Design review of the part built by this model. Coordinates are the model's own, in mm. A direction names the side the tool comes from. Give positions to 0.01 mm unless a question says otherwise; leave off trailing zeros. Write each loop counter-clockwise with the first axis right and the second up, starting at its lowest first coordinate (ties: lowest second). Pieces come first, ordered by that corner, then holes. Notation, with made-up numbers: M 71.25,64 L 114.25,64 A19 ccw 114.25,96 Z; hole C 74,48 d9. An arc over 180 degrees is marked long. Answer in a Markdown table with one row per item.
```python
from build123d import *

# Parameters (mm, degrees)
SKETCH1_W                             = 57.5
SKETCH1_H                             = 35.8
BASE_EXTRUSION_DEPTH                  = 0.79375
SKETCH2_R                             = 0.25
PIR_MOUNTING_HOLES_DEPTH              = 36.158249943
SKETCH3_R                             = 0.555
CONNECTOR_MOUNTING_HOLE_DEPTH         = 36.158249943
CONNECTOR_MOUNTING_HOLE_PATTERN_COUNT = 5
CONNECTOR_MOUNTING_HOLE_PATTERN_PITCH = 2.5
SKETCH4_W                             = 25
SKETCH4_H                             = 9.9
LED_DRIVER_CLEARANCE_CUT_DEPTH        = 36.158249943
LED_DRIVER_CLEARANCE_CUT_FILLETS_R    = 3
CORNER_CUTOUT_DEPTH                   = 36.158249943
SKETCH7_R                             = 1.1
MOUNTING_SCREW_HOLES_DEPTH            = 36.158249943


with BuildPart() as part:
    # Sketch1 → Base Extrusion (new body)
    with BuildSketch(Plane(origin=(0, 0, 0), x_dir=(1, 0, 0), z_dir=(0, 1, 0))):
        with Locations((-1.5, 0)):
            Rectangle(SKETCH1_W, SKETCH1_H)
    extrude(amount=BASE_EXTRUSION_DEPTH)

    # Sketch2 → PIR Mounting Holes (cut, through all)
    with BuildSketch(Plane(origin=(0, 0.79375, 0), x_dir=(1, 0, 0), z_dir=(0, 1, 0))):
        with Locations(Location((1.796051224, -1.796051224, 0), (0, 0, 270))):
            Circle(SKETCH2_R)
        with Locations(Location((1.796051224, 1.796051224, 0), (0, 0, 270))):
            Circle(SKETCH2_R)
        with Locations(Location((-1.796051224, -1.796051224, 0), (0, 0, 270))):
            Circle(SKETCH2_R)
    extrude(amount=-PIR_MOUNTING_HOLES_DEPTH, mode=Mode.SUBTRACT)

    # Sketch3 → Connector Mounting Hole (cut, through all)
    with BuildSketch(Plane(origin=(0, 0.79375, 0), x_dir=(1, 0, 0), z_dir=(0, 1, 0))):
        with Locations(Location((-25.75, 5, 0), (0, 0, 270))):
            Circle(SKETCH3_R)
    connector_mounting_hole = extrude(amount=-CONNECTOR_MOUNTING_HOLE_DEPTH, mode=Mode.SUBTRACT)

    # Connector Mounting Hole Pattern: Connector Mounting Hole ×5
    with Locations(*[(0, 0, i * CONNECTOR_MOUNTING_HOLE_PATTERN_PITCH) for i in range(1, CONNECTOR_MOUNTING_HOLE_PATTERN_COUNT)]):
        add(connector_mounting_hole, mode=Mode.SUBTRACT)

    # Sketch4 → LED Driver Clearance Cut (cut, through all)
    with BuildSketch(Plane.XZ):
        with Locations((-1.5, -12.95)):
            Rectangle(SKETCH4_W, SKETCH4_H)
    extrude(amount=-LED_DRIVER_CLEARANCE_CUT_DEPTH, mode=Mode.SUBTRACT)

    # LED Driver Clearance Cut Fillets
    led_driver_clearance_cut_fillets_edges = [part.edges().sort_by_distance(p)[0] for p in [
        (-14, 0.396875, -8),
        (11, 0.396875, -8),
    ]]
    fillet(led_driver_clearance_cut_fillets_edges, radius=LED_DRIVER_CLEARANCE_CUT_FILLETS_R)

    # Sketch5 → Corner Cutout (cut, through all)
    with BuildSketch(Plane(origin=(0, 0.79375, 0), x_dir=(1, 0, 0), z_dir=(0, 1, 0))):
        with BuildLine():
            Line((-30.25, 11), (-27.5, 11))
            ThreePointArc((-27.5, 11), (-25.697080654, 11.602192287), (-24.617964056, 13.167012113))
            Line((-24.617964056, 13.167012113), (-23.25, 17.9))
            Line((-23.25, 17.9), (-30.25, 17.9))
            Line((-30.25, 17.9), (-30.25, 11))
        make_face()
        with BuildLine():
            Line((20.25, 17.9), (21.617964056, 13.167012113))
            ThreePointArc((21.617964056, 13.167012113), (22.697080654, 11.602192287), (24.5, 11))
            Line((24.5, 11), (27.25, 11))
            Line((27.25, 11), (27.25, 17.9))
            Line((27.25, 17.9), (20.25, 17.9))
        make_face()
    corner_cutout = extrude(amount=-CORNER_CUTOUT_DEPTH, mode=Mode.SUBTRACT)

    # Corner Cut Mirror: Corner Cutout across plane
    add(corner_cutout.mirror(Plane.XY), mode=Mode.SUBTRACT)

    # Sketch7 → Mounting Screw Holes (cut, through all)
    with BuildSketch(Plane(origin=(0, 0.79375, 0), x_dir=(1, 0, 0), z_dir=(0, 1, 0))):
        with Locations(Location((-19.5, 14, 0), (0, 0, 270))):
            Circle(SKETCH7_R)
        with Locations(Location((-19.5, -14, 0), (0, 0, 270))):
            Circle(SKETCH7_R)
        with Locations(Location((16.5, -14, 0), (0, 0, 270))):
            Circle(SKETCH7_R)
        with Locations(Location((16.5, 14, 0), (0, 0, 270))):
            Circle(SKETCH7_R)
    extrude(amount=-MOUNTING_SCREW_HOLES_DEPTH, mode=Mode.SUBTRACT)


solid = part.part
```
1) For faces 4 (the face through (15.426, 0.402, 13.762)), 5 (the face through (10.1, 0.4, -8.86)), list the 3-axis set-ups (+Z, -Z, +X, -X, +Y, -Y) from which the entire face can be reached by the end or side of a thin tool; tool diameter is ignored.
Geometry says:
| item | result |
|---|---|
| face 4 | +Y, -Y |
| face 5 | -Z, +Y, -Y |
2) To check wall thickness, follow probe 1 along Z at (x, y) = (-3, 0.3); probe 2 along Z at (x, y) = (-20, 0.4); probe 3 along X at (y, z) = (0.3, -5) (3 decimals). State the ranges of each line that lie inside material, in increasing order. Write a range as [from, to].
Geometry says:
| item | result |
|---|---|
| probe 1 | [-8, 17.9] |
| probe 2 | [-17.9, -14.98], [-13.02, 13.02], [14.98, 17.9] |
| probe 3 | [-30.25, -26.305], [-25.195, 27.25] |
3) Add section C-C (z = -14). Write out the cut boundary in (x, y).
Geometry says:
| item | result |
|---|---|
| outline | M -24.38,0 L -20.6,0 L -20.6,0.79 L -24.38,0.79 Z; M -18.4,0 L -14,0 L -14,0.79 L -18.4,0.79 Z; M 11,0 L 15.4,0 L 15.4,0.79 L 11,0.79 Z; M 17.6,0 L 21.38,0 L 21.38,0.79 L 17.6,0.79 Z |
4) Add section D-D (y = 0.55). Count the separate pieces of the cut face and the enclosed holes in it, and give its area (3 significant figures).
Geometry says:
| item | result |
|---|---|
| separate pieces | 1 |
| enclosed holes | 12 |
| area | 1,630 mm^2 |
5) Add section A-A (x = 16.5). Write out the cut boundary in (y, z).
Geometry says:
| item | result |
|---|---|
| outline | M 0,-17.9 L 0.79,-17.9 L 0.79,-15.1 L 0,-15.1 Z; M 0,-12.9 L 0.79,-12.9 L 0.79,12.9 L 0,12.9 Z; M 0,15.1 L 0.79,15.1 L 0.79,17.9 L 0,17.9 Z |
6) Add section B-B (z = 0). Write out the cut boundary in (x, y) (3 decimals), and give its area (3 significant figures).
Geometry says:
| item | result |
|---|---|
| outline | M -30.25,0 L -26.305,0 L -26.305,0.794 L -30.25,0.794 Z; M -25.195,0 L 27.25,0 L 27.25,0.794 L -25.195,0.794 Z |
| area | 44.8 mm^2 |
7) Insertion check: P1, Ø1.5, axis at x = 4, z = -9.5, coming from the -Y side. The pin has a flat end and moves straight along its axis. Give the tip position at first contact, or say it passes through.
Geometry says:
| item | result |
|---|---|
| P1 | through |
8) The part is to be moulded in two halves that separate along X. For faces 1 (the face through (-23.944, 0.402, 15.5)), 2 (the face through (-2, 0.794, 4)), 3 (the face through (-25.2, 0.4, -5.07)), say which applies: released by +X, released by -X, zero draft, split by the parting line, or undercut.
Geometry says:
| item | result |
|---|---|
| face 1 | released by -X |
| face 2 | zero draft |
| face 3 | undercut |
